Geometry: see drawing. Coordinates: mm, zero at the bounding-box minimum. A direction names the side the tool comes from. Round coordinates to 2 decimals unless told otherwise and drop trailing zeros. Write each loop counter-clockwise with the first axis right and the second up, starting at its lowest first coordinate (ties: lowest second). Pieces come first, ordered by that corner, then holes. Notation, with made-up numbers: (50, 82) -> (92, 82) arc R9 cw to (92, 92) -> close; hole circle Ø9 at (74.25, -8). An arc over 180 degrees is marked (long way). Write item = value, one per line.
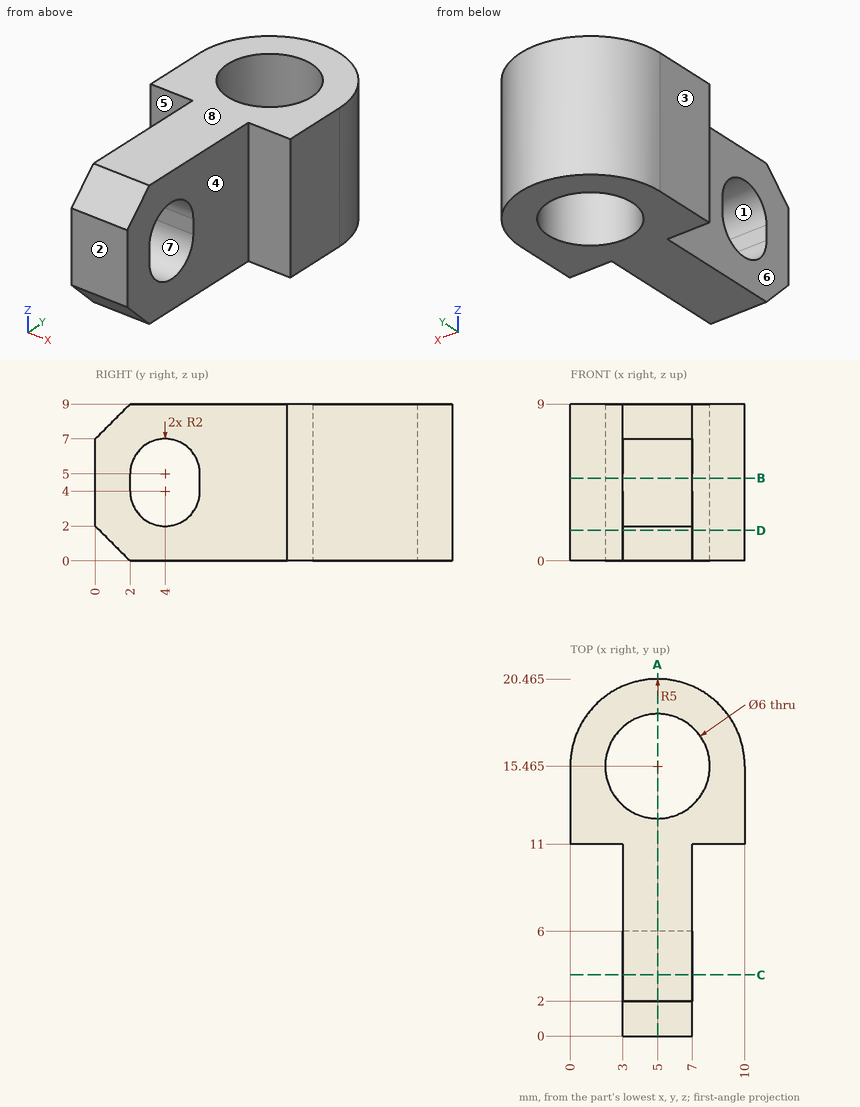
1) First-contact query: P1, Ø2.5, axis at y = 6.5, z = 3.5, coming from the +X side; P2, Ø1, axis at x = 6, y = 14, coming from the -Z side; P3, Ø2, axis at y = 8.5, z = 7.5, coming from the -X side; P4, Ø1.5, axis at x = 2, z = 5.5, coming from the -Y side. Flat tips, straight axial feed; report the tip coordinate or a pass-through.
Solutions:
P1 = 7
P2 = through
P3 = 3
P4 = 11
2) Line query: L1, parallel to Z at x = 4.75, y = 4; L2, parallel to Y at x = 5, z = 3.5 (1 decimal); L3, parallel to X at y = 14, z = 7.5. Output: solid intervals per line, ascending. Write a range as from..to.
Solutions:
L1 = 0..2, 7..9
L2 = 0..2.1, 5.9..12.5, 18.5..20.5
L3 = 0..2.38, 7.62..10
3) Cut plane D-D (z = 1.75). Return the cut outline in (x, y) (3 decimals).
Solutions:
outline = (0, 11) -> (3, 11) -> (3, 0.25) -> (7, 0.25) -> (7, 11) -> (10, 11) -> (10, 15.465) arc R5 ccw to (0, 15.465) -> close; hole circle Ø6 at (5, 15.465)
4) Draft query along Z for the marked faces 6, 7 and 8. Return one class per face: +Z half, -Z half, draft (parallel to the pull), parting line (faces both ways), or undercut.
Solutions:
face_6 = draft
face_7 = undercut
face_8 = +Z half
5) Cut plane A-A (x = 5). Return the cut outline in (y, z) (3 decimals), and give its area (3 significant figures).
Solutions:
outline = (0, 2) -> (2, 0) -> (12.465, 0) -> (12.465, 9) -> (2, 9) -> (0, 7) -> close; (18.465, 0) -> (20.465, 0) -> (20.465, 9) -> (18.465, 9) -> close; hole (2, 4) arc R2 ccw to (6, 4) -> (6, 5) arc R2 ccw to (2, 5) -> close
area = 110 mm^2
6) Access query for the marked faces 1, 2, 3, 4 and 5. Directions: +Z, -Z, +X, -X, +Y, -Y. A direction counts if a zero-diameter tool reaches every point of the face in a straight line with its end or side. Return the directions, or none.
Solutions:
face_1 = +X, -X
face_2 = +Z, -Z, +X, -X, -Y
face_3 = +Z, -Z, -X, +Y, -Y
face_4 = +Z, -Z, +X, -Y
face_5 = +Z, -Z, -X, -Y
7) Cut plane B-B (z = 4.75). Return the cut outline in (x, y) (3 decimals).
Solutions:
outline = (0, 11) -> (3, 11) -> (3, 6) -> (7, 6) -> (7, 11) -> (10, 11) -> (10, 15.465) arc R5 ccw to (0, 15.465) -> close; (3, 0) -> (7, 0) -> (7, 2) -> (3, 2) -> close; hole circle Ø6 at (5, 15.465)
8) Cut plane C-C (y = 3.5). Return the cut outline in (x, z), and give its area (3 significant figures).
Solutions:
outline = (3, 0) -> (7, 0) -> (7, 2.06) -> (3, 2.06) -> close; (3, 6.94) -> (7, 6.94) -> (7, 9) -> (3, 9) -> close
area = 16.5 mm^2
